```python
from build123d import *

# Parameters (mm, degrees)
F0_W     = 19.7
F0_H     = 111
F1_DEPTH = 1.3
F3_DEPTH = 10
F4_W     = 19.7
F4_H     = 21
F5_DEPTH = 10
F7_DEPTH = 21


with BuildPart() as f1:
    # F0 (on Top) → F1 (new body)
    with BuildSketch(Plane.XY):
        with Locations((9.85, 55.5)):
            Rectangle(F0_W, F0_H)
    extrude(amount=F1_DEPTH)

    # F2 (on face) → F3 (join)
    with BuildSketch(Plane.XY.offset(1.3)):
        Polygon((12.625, 98.1), (7.075, 98.1), (3.075, 97.1), (3.075, 13.9), (7.075, 12.9), (12.625, 12.9), (16.625, 13.9), (16.625, 97.1), align=None)
    extrude(amount=F3_DEPTH)

    # F4 (on face) → F5 (join)
    with BuildSketch(Plane.XY.offset(1.3)):
        with Locations((9.85, 55.5)):
            Rectangle(F4_W, F4_H)
    extrude(amount=F5_DEPTH)

    # F6 (on face) → F7 (join, through all)
    with BuildSketch(Plane(origin=(0, 66, 0), x_dir=(-1, 0, 0), z_dir=(0, 1, 0))):
        Polygon((-16.575, 11.3), (-3.075, 11.3), (-4.125, 16.5472850204), (-15.625, 16.5472850204), align=None)
    extrude(amount=-F7_DEPTH)


solid = f1.part
```
For this review, take the finished solid that the model builds, in its own axes (mm). A direction names the side the tool comes from. Coordinates: 2 decimals unless noted, no trailing zeros. Write each loop counter-clockwise with the first axis right and the second up, starting at its lowest first coordinate (ties: lowest second). Pieces come first, ordered by that corner, then holes. Notation, with made-up numbers: (41, 82) - (98, 82) arc R25 cw to (98, 117) - close; hole circle Ø4 at (77.25, 56.5). An arc over 180 degrees is marked (long way). Answer in a Markdown table with one row per item. Add a question column.
Q1. We need section C-C, the plane z = 7. State the section outline as (x, y) points (3 decimals).
Q2. Tool access review of faces 1 (the flat face through (10, 66, 14)), 2 (the flat face through (14.597, 13.393, 6.23)), 3 (the flat face through (2, 66, 6)), 4 (the flat face through (2, 45, 6)): name each direction out of +Z, -Z, +X, -X, +Y, -Y from which nothing blocks a thin tool from reaching the whole face with its end or side.
Q3. We need section D-D, the plane y = 55.5. State the section outline as (x, z) points (3 decimals).
Q4. We need section A-A, the plane y = 42. State the section outline as (x, z) points (3 decimals).
Q5. For probe 1 along X at (y, z) = (28.5, 1.75) (3 decimals); probe 2 along Y at (x, z) = (17.75, 3); probe 3 along Z at (x, y) = (14.5, 78), list the stretches that pass through material, from the lowest coordinate up.
Q6. We need section B-B, the plane x = 11.25. State the section outline as (y, z) points, and give its area (3 significant figures).
Q7. Draft analysis for pull direction X (two halves, no side actions). For faces 5 (the flat face through (0, 55, 4)), 6 (the flat face through (14.653, 97.593, 6.23)), 7 (the flat face through (10, 12.9, 6)), state which applies: +X half, -X half, draft (parallel to the pull), parting line (faces both ways), or undercut.
Q8. For P1, Ø6, axis at x = 12, z = 14.5, coming from the +Y side; P2, Ø4, axis at x = 7, z = 9, coming from the +Y side; P3, Ø0.9, axis at x = 18, z = 6.5, coming from the -Y side, all flat-tipped, find the tip position at first contact; note any pin that passes through.
Answer list:
| question | item | result |
|---|---|---|
| 1 | outline | (0, 45) - (3.075, 45) - (3.075, 13.9) - (7.075, 12.9) - (12.625, 12.9) - (16.625, 13.9) - (16.625, 45) - (19.7, 45) - (19.7, 66) - (16.625, 66) - (16.625, 97.1) - (12.625, 98.1) - (7.075, 98.1) - (3.075, 97.1) - (3.075, 66) - (0, 66) - close |
| 2 | face 1 | +Z, +X, -X, +Y |
| 2 | face 2 | +Z, +X, -Y |
| 2 | face 3 | +Z, -X, +Y |
| 2 | face 4 | +Z, -X, -Y |
| 3 | outline | (0, 0) - (19.7, 0) - (19.7, 11.3) - (16.575, 11.3) - (15.625, 16.547) - (4.125, 16.547) - (3.075, 11.3) - (0, 11.3) - close |
| 4 | outline | (0, 0) - (19.7, 0) - (19.7, 1.3) - (16.625, 1.3) - (16.625, 11.3) - (3.075, 11.3) - (3.075, 1.3) - (0, 1.3) - close |
| 5 | probe 1 | x = 3.075 to 16.625 |
| 5 | probe 2 | y = 45 to 66 |
| 5 | probe 3 | z = 0 to 11.3 |
| 6 | outline | (0, 0) - (111, 0) - (111, 1.3) - (98.1, 1.3) - (98.1, 11.3) - (66, 11.3) - (66, 16.55) - (45, 16.55) - (45, 11.3) - (12.9, 11.3) - (12.9, 1.3) - (0, 1.3) - close |
| 6 | area | 1,110 mm2 |
| 7 | face 5 | -X half |
| 7 | face 6 | +X half |
| 7 | face 7 | draft |
| 8 | P1 | stops at y = 66 |
| 8 | P2 | stops at y = 98.1 |
| 8 | P3 | stops at y = 45 |
